Autodesk Inventor part; units mm, degrees
ref_plane "YZ Plane" through (0, 0, 0) normal (1, 0, 0) x (0, 1, 0)
ref_plane "XZ Plane" through (0, 0, 0) normal (0, 1, 0) x (-1, 0, 0)
ref_plane "XY Plane" through (0, 0, 0) normal (0, 0, 1) x (1, 0, 0)
sketch "Sketch1" plane through (0, 0, 0) normal (0, 1, 0) x (-1, 0, 0)
  line L0 (0, 0) -> (53.575, 0)
  line L1 (53.575, 0) -> (53.575, -50.8)
  line L2 (53.575, -50.8) -> (0, -50.8)
  line L3 (0, -50.8) -> (0, 0)
  line L4 (10, 0) -> (10, -50.8)
  arc A0 (30.4, -35.8017) -> (30.4, -42.1517) centre (30.4, -38.9767) ccw
  arc A1 (40.4, -42.1517) -> (40.4, -35.8017) centre (40.4, -38.9767) ccw
  line L5 (30.4, -35.8017) -> (40.4, -35.8017)
  line L6 (40.4, -42.1517) -> (30.4, -42.1517)
  line L7 (-7.5059, -25.4) -> (68.7329, -25.4)
  arc A2 (30.4, -8.6483) -> (30.4, -14.9983) centre (30.4, -11.8233) ccw
  arc A3 (40.4, -14.9983) -> (40.4, -8.6483) centre (40.4, -11.8233) ccw
  line L8 (30.4, -14.9983) -> (40.4, -14.9983)
  line L9 (40.4, -8.6483) -> (30.4, -8.6483)
  dimension "d0" = 50.8
  dimension "d2" = 10
  dimension "d3" = 6.35
  dimension "d4" = 6.35
  dimension "d6" = 10
  dimension "d7" = 20.4
  dimension "d8" = 13.175
  dimension "d9" = 25.4
extrude "Extrusion1" add sketch "Sketch1" along normal blind 10
sketch "Sketch2" plane through (0, 10, 0) normal (0, 1, 0) x (1, 0, 0)
  line L0 (0, 50.8) -> (-53.575, 50.8)
  line L1 (0, 0) -> (-10, 0)
  line L2 (-10, 0) -> (-10, 50.8)
  line L3 (-10, 50.8) -> (0, 50.8)
  line L4 (0, 50.8) -> (0, 0)
  dimension "d12" = 10
extrude "Extrusion2" add sketch "Sketch2" along normal blind 36
sketch "Sketch3" plane through (0, 0, 0) normal (1, 0, 0) x (0, 0, -1)
  line L0 (0, 10) -> (50.8, 10)
  circle A0 centre (8, 28) radius 1.42
  circle A1 centre (42.8, 28) radius 1.42
  line L1 (50.8, 0) -> (50.8, 46)
  line L2 (0, 0) -> (0, 46)
  line L3 (0, 0) -> (50.8, 0)
  line L4 (50.8, 0) -> (50.8, 46)
  line L5 (0, 46) -> (50.8, 46)
  line L6 (0, 0) -> (0, 46)
  arc A2 (20.4, 24.5) -> (20.4, 16.5) centre (20.4, 20.5) ccw
  arc A3 (30.4, 16.5) -> (30.4, 24.5) centre (30.4, 20.5) ccw
  line L7 (20.4, 24.5) -> (30.4, 24.5)
  line L8 (20.4, 16.5) -> (30.4, 16.5)
  line L9 (20.4, 20.5) -> (25.4, 20.5)
  point P0 (50.8, 23)
  point P1 (25.4, 10)
  dimension "d15" = 2.84
  dimension "d16" = 2.84
  dimension "d17" = 34.8
  dimension "d18" = 0
  dimension "d19" = 18
  dimension "d20" = 8
  dimension "d21" = 8
  dimension "d22" = 50.8
  dimension "d35" = 8
  dimension "d36" = 8
  dimension "d37" = 0
  dimension "d38" = 10
  dimension "d39" = 5
  dimension "d40" = 25.4
  dimension "d41" = 10.5
extrude "Extrusion3" cut sketch "Sketch3" against normal blind 36 contours A0 | A1 | L7 A3 L8 A2
sketch "Sketch4" plane through (0, 10, 0) normal (0, 1, 0) x (1, 0, 0)
  arc A0 (-40.4, 42.1517) -> (-40.4, 35.8017) centre (-40.4, 38.9767) ccw
  arc A1 (-40.4, 43.9767) -> (-40.4, 33.9767) centre (-40.4, 38.9767) ccw
  arc A2 (-30.4, 35.8017) -> (-30.4, 42.1517) centre (-30.4, 38.9767) ccw
  arc A3 (-30.4, 33.9767) -> (-30.4, 43.9767) centre (-30.4, 38.9767) ccw
  line L0 (-10, 0) -> (-10, 50.8)
  line L1 (-10, 50.8) -> (-53.575, 50.8)
  line L2 (-53.575, 50.8) -> (-53.575, 0)
  line L3 (-53.575, 0) -> (-10, 0)
  line L4 (-40.4, 14.9983) -> (-30.4, 14.9983)
  arc A4 (-30.4, 8.6483) -> (-30.4, 14.9983) centre (-30.4, 11.8233) ccw
  line L5 (-30.4, 8.6483) -> (-40.4, 8.6483)
  arc A5 (-40.4, 14.9983) -> (-40.4, 8.6483) centre (-40.4, 11.8233) ccw
  line L6 (-40.4, 42.1517) -> (-30.4, 42.1517)
  arc A6 (-30.4, 35.8017) -> (-30.4, 42.1517) centre (-30.4, 38.9767) ccw
  line L7 (-30.4, 35.8017) -> (-40.4, 35.8017)
  arc A7 (-40.4, 42.1517) -> (-40.4, 35.8017) centre (-40.4, 38.9767) ccw
  arc A8 (-40.4, 16.8233) -> (-40.4, 6.8233) centre (-40.4, 11.8233) ccw
  arc A9 (-30.4, 6.8233) -> (-30.4, 16.8233) centre (-30.4, 11.8233) ccw
  line L8 (-30.4, 6.8233) -> (-40.4, 6.8233)
  line L9 (-40.4, 16.8233) -> (-30.4, 16.8233)
  line L10 (-30.4, 33.9767) -> (-40.4, 33.9767)
  line L11 (-40.4, 43.9767) -> (-30.4, 43.9767)
  point P0 (0, 0)
  dimension "d25" = 10
  dimension "d26" = 10
  dimension "d27" = 10
  dimension "d28" = 10
extrude "Extrusion4" cut sketch "Sketch4" against normal blind 6 contours L6 A2 L7 A0 | L11 A3 L10 A1 | L4 A4 L5 A5 | L9 A9 L8 A8
sketch "Sketch5" plane through (0, 0, 0) normal (1, 0, 0) x (0, 0, -1)
  circle A0 centre (42.8, 28) radius 1.42
  circle A1 centre (8, 28) radius 1.42
  line L0 (0, 0) -> (50.8, 0)
  line L1 (50.8, 0) -> (50.8, 46)
  line L2 (0, 46) -> (50.8, 46)
  line L3 (0, 0) -> (0, 46)
  circle A2 centre (8, 28) radius 3
  circle A3 centre (42.8, 28) radius 1.42
  circle A4 centre (42.8, 28) radius 3
  dimension "d31" = 6
  dimension "d32" = 6
extrude "Extrusion5" cut sketch "Sketch5" against normal blind 5 contours A1 | A2 | A4
equation "\"d4\" = d3"
equation "\"d9\" = 0.5 * d0"
equation "\"d12\" = d2"
equation "\"d16\" = d15"
equation "\"d20\" = -0.5 * d17 + 0.5 * d22"
equation "\"d36\" = d35"
equation "\"d39\" = 0.5 * d38"
equation "\"d26\" = d25"
equation "\"d27\" = d25"
equation "\"d28\" = d25"
equation "\"d32\" = d31"
properties part number "Actuator Stage End Cap"
Can you work these out from the model? Positions are in its coordinate system, mm. A direction names the side the tool comes from. Round coordinates to 2 decimals unless told otherwise and drop trailing zeros. Loops run counter-clockwise (first coordinate to the right, second up) from the corner with the lowest first, then second, coordinate; pieces in that order, holes last. Notation, with made-up numbers: M 22,38.5 L 55,38.5 A25 cw 55,65.5 Z; hole C 28,35 d4. An arc over 180 degrees is marked long. Write item = value, one per line. Start each with the question number.
(1) I need wall thicknesses on line 1 along Y through (x, z) = (-6.35, -8); line 2 along Y through (x, z) = (-2.9, -42.8); line 3 along X through (y, z) = (10.5, -22). Which ranges of each line are inside material? Lowest first, please.
(2) Suppose I cut it at A-A on x = -37. Write out the boundary of the cut face in (y, z), plus the area to 3 significant figures.
(3) If we mould it in two halves opening along Z, with no side actions, what happens to faces 1 (the face through (-35, 2, -35.802)), 2 (the face through (-26, 0, -25))? For each: released by +Z, released by -Z, zero draft, split by the parting line, or undercut.
(4) I'm going to push flat-ended pins straight in: P1, Ø13, axis at x = -32, z = -17.5, coming from the +Y side; P2, Ø10, axis at x = -22.5, z = -13.5, coming from the -Y side; P3, Ø4, axis at y = 28.5, z = -6.5, coming from the -X side; P4, Ø1.8, axis at y = 28.5, z = -7, coming from the +X side. Where does each tip first touch, or does it pass through?
(5) Which directions (+Z, -Z, +X, -X, +Y, -Y) give clear straight access to the entire face, cutting with the end or side of a thin tool? Please do faces 3 (the face through (-35, 7, -6.823)), 4 (the face through (-5, 27, -41)), 5 (the face through (-27.226, 1.972, -39.047)), 6 (the face through (-10, 28, -25)).
(6) Suppose I cut it at C-C on y = 28. Write out the boundary of the cut face in (x, z), plus the area to 3 significant figures.
(7) Suppose I cut it at D-D on z = -18.5. Write out the boundary of the cut face in (x, y) (3 decimals).
(8) Suppose I cut it at B-B on y = 20.5. Write out the boundary of the cut face in (x, z).
Answer block:
q1.line_1 = 0 to 26.58, 29.42 to 46
q1.line_2 = 0 to 25, 31 to 46
q1.line_3 = -10 to 0
q2.outline = M 0,-50.8 L 10,-50.8 L 10,-43.98 L 4,-43.98 L 4,-42.15 L 0,-42.15 Z; M 0,-35.8 L 4,-35.8 L 4,-33.98 L 10,-33.98 L 10,-16.82 L 4,-16.82 L 4,-15 L 0,-15 Z; M 0,-8.65 L 4,-8.65 L 4,-6.82 L 10,-6.82 L 10,0 L 0,0 Z
q2.area = 337 mm²
q3.face_1 = undercut
q3.face_2 = zero draft
q4.P1 = 10
q4.P2 = 0
q4.P3 = -10
q4.P4 = -5
q5.face_3 = +Y
q5.face_4 = +X
q5.face_5 = +Y, -Y
q5.face_6 = +Z, -Z, -X, +Y
q6.outline = M -10,-50.8 L 0,-50.8 L 0,-45.8 L -5,-45.8 L -5,-44.22 L -10,-44.22 Z; M -10,-41.38 L -5,-41.38 L -5,-39.8 L 0,-39.8 L 0,-11 L -5,-11 L -5,-9.42 L -10,-9.42 Z; M -10,-6.58 L -5,-6.58 L -5,-5 L 0,-5 L 0,0 L -10,0 Z
q6.area = 420 mm²
q7.outline = M -53.575,0 L 0,0 L 0,16.98 L -10,16.98 L -10,10 L -53.575,10 Z; M -10,24.02 L 0,24.02 L 0,46 L -10,46 Z
q8.outline = M -10,-50.8 L 0,-50.8 L 0,-34.4 L -10,-34.4 Z; M -10,-16.4 L 0,-16.4 L 0,0 L -10,0 Z
